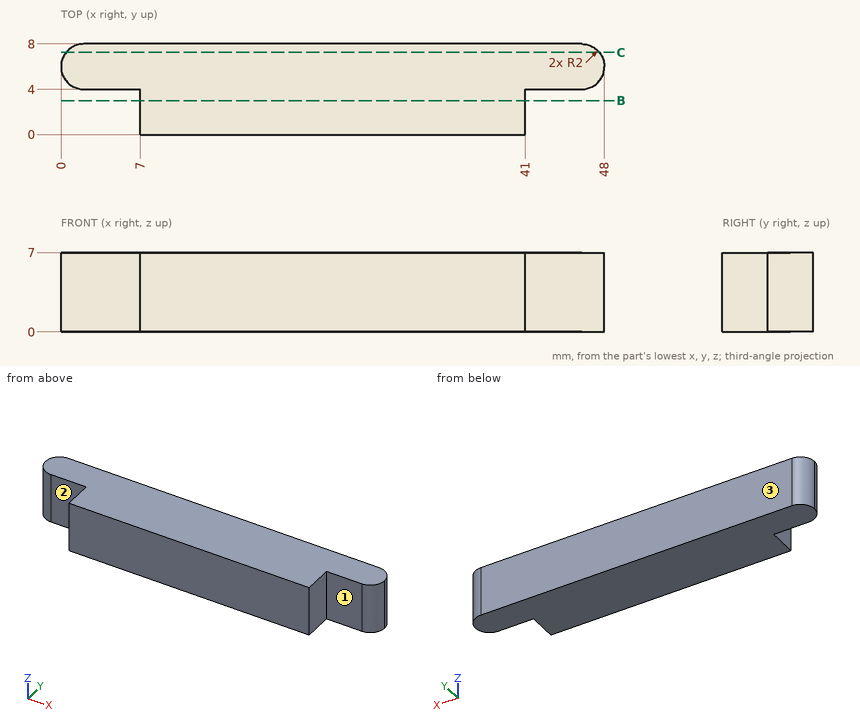
Design review of the part shown in the three views and the two pictorial views. Dimensions are in mm from the part's minimum x, y and z. A direction names the side the tool comes from. Give positions to 0.01 mm unless a question says otherwise; leave off trailing zeros. Loops run counter-clockwise (first coordinate to the right, second up) from the corner with the lowest first, then second, coordinate; pieces in that order, holes last. Notation, with made-up numbers: M 68,-38 L 80,-38 A15 cw 80,-17 Z; hole C 82.5,39.25 d6. An arc over 180 degrees is marked long. Write item = value, one per line.
Q1. Insertion check: pin 1 (1.5 mm diameter, centred on x = 4.5, z = 4, fed in from -Y); pin 2 (1.2 mm diameter, centred on y = 2, z = 5, fed in from -X); pin 3 (1 mm diameter, centred on y = 5, z = 4.5, fed in from +X). Each pin has a flat end and moves straight along its axis. Give the tip position at first contact, or say it passes through.
Output values:
pin_1 = 4
pin_2 = 7
pin_3 = 47.94
Q2. To check wall thickness, follow line 1 (Y direction, x = 45.5, z = 4.75); line 2 (X direction, y = 3, z = 5.25); line 3 (X direction, y = 7.75, z = 0.5). State the ranges of each line that lie inside material, in increasing order. Write a range as [from, to].
Output values:
line_1 = [4, 8]
line_2 = [7, 41]
line_3 = [1.03, 46.97]
Q3. We need section B-B (y = 3). Give the boundary of the cut face in (x, z).
Output values:
outline = M 7,0 L 41,0 L 41,7 L 7,7 Z
Q4. For the marked faces 1, 2 and 3, list the 3-axis set-ups (+Z, -Z, +X, -X, +Y, -Y) from which the entire face can be reached by the end or side of a thin tool; tool diameter is ignored.
Output values:
face_1 = +Z, -Z, +X, -Y
face_2 = +Z, -Z, -X, -Y
face_3 = +Z, -Z, +X, -X, +Y
Q5. We need section C-C (y = 7.25). Give the boundary of the cut face in (x, z), plus the area to 3 significant figures.
Output values:
outline = M 0.44,0 L 47.56,0 L 47.56,7 L 0.44,7 Z
area = 330 mm^2
